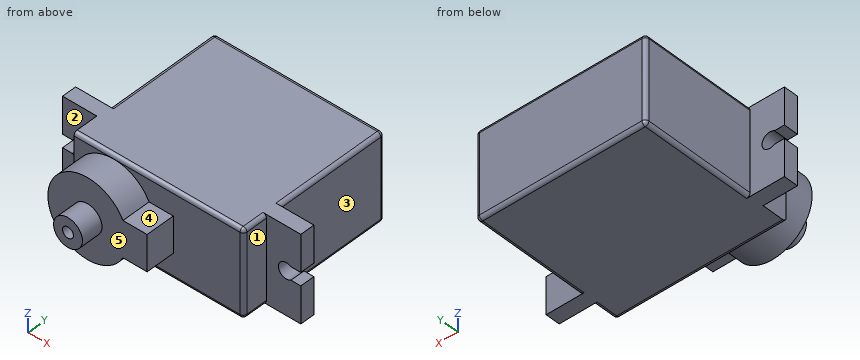
Autodesk Inventor part; units mm, degrees
ref_plane "YZ Plane" through (0, 0, 0) normal (1, 0, 0) x (0, 1, 0)
ref_plane "XZ Plane" through (0, 0, 0) normal (0, 1, 0) x (-1, 0, 0)
ref_plane "XY Plane" through (0, 0, 0) normal (0, 0, 1) x (1, 0, 0)
sketch "Sketch1" plane through (0, 0, 0) normal (0, 0, 1) x (1, 0, 0)
  line L0 (0, 0) -> (23.5, 0)
  line L1 (23.5, 0) -> (23.5, -21.5)
  line L2 (23.5, -21.5) -> (0, -21.5)
  line L3 (0, -21.5) -> (0, 0)
  dimension "d0" = 23.5
  dimension "d1" = 21.5
extrude "Extrusion1" add sketch "Sketch1" against normal blind 12
sketch "Sketch2" plane through (0, 0, 0) normal (0, 0, 1) x (1, 0, 0)
  line L0 (0, 0) -> (23.5, 0)
  line L1 (0, -21.5) -> (0, 0)
  line L2 (23.5, 0) -> (23.5, -21.5)
  line L3 (-4.75, -16) -> (28.25, -16)
  line L4 (28.25, -16) -> (28.25, -18)
  line L5 (28.25, -18) -> (-4.75, -18)
  line L6 (-4.75, -18) -> (-4.75, -16)
  dimension "d4" = 16
  dimension "d5" = 4.75
  dimension "d6" = 4.75
  dimension "d7" = 2
extrude "Extrusion2" add sketch "Sketch2" against normal blind 12 contours L3 L2 L5 L1 | L1 L5 L6 L3 | L3 L4 L5 L2
sketch "Sketch3" plane through (0, -21.5, 0) normal (0, -1, 0) x (1, 0, 0)
  line L0 (0, 0) -> (0, -12)
  circle A0 centre (5.5, -6) radius 5.5
  dimension "d10" = 5.5
  dimension "d11" = 11
extrude "Extrusion3" add sketch "Sketch3" along normal blind 4
sketch "Sketch4" plane through (5.5, -25.5, -6) normal (0, -1, 0) x (1, 0, 0)
  circle A0 centre (0, 0) radius 5.5
  line L0 (4.8288, 2.5) -> (8.25, 2.5)
  line L1 (8.25, 2.5) -> (8.25, -2.5)
  line L2 (8.25, -2.5) -> (4.8288, -2.5)
  line L3 (4.8288, -2.5) -> (4.8288, 2.5)
  point P0 (-5.5, 6)
  point P1 (8.25, 0)
  dimension "d15" = 5
  dimension "d17" = 8.25
extrude "Extrusion4" add sketch "Sketch4" against normal blind 4 contours A0 L2 L3 L0 | A0 L0 L1 L2 picked at (4.9626, -0.5673)
sketch "Sketch5" plane through (0, -25.5, 0) normal (0, -1, 0) x (1, 0, 0)
  arc A0 (10.399, -3.5) -> (10.399, -8.5) centre (5.5, -6) ccw
  circle A1 centre (5.5, -6) radius 2
  point P0 (0, 0)
  dimension "d20" = 4
extrude "Extrusion5" add sketch "Sketch5" along normal blind 3
sketch "Sketch6" plane through (-4.75, -18, 0) normal (0, -1, 0) x (1, 0, 0)
  line L0 (4.75, 0) -> (4.75, -12)
  line L1 (0, 0) -> (0, -12)
  line L2 (28.25, -12) -> (28.25, 0)
  line L3 (33, -12) -> (28.25, -12)
  line L4 (33, 0) -> (33, -12)
  line L5 (33, 0) -> (28.25, 0)
  circle A0 centre (2, -6) radius 1.1
  circle A1 centre (31, -6) radius 1.1
  line L6 (-3.3152, -5.1) -> (1.5271, -5.1)
  line L7 (1.5271, -5.1) -> (1.5271, -6.9)
  line L8 (1.5271, -6.9) -> (-3.3152, -6.9)
  line L9 (-3.3152, -6.9) -> (-3.3152, -5.1)
  line L10 (31.5226, -5.1) -> (37.6277, -5.1)
  line L11 (37.6277, -5.1) -> (37.6277, -6.9)
  line L12 (37.6277, -6.9) -> (31.5226, -6.9)
  line L13 (31.5226, -6.9) -> (31.5226, -5.1)
  point P0 (4.75, -6)
  point P1 (1.5271, -6)
  point P2 (28.25, -6)
  point P3 (31.5226, -6)
  dimension "d24" = 2.2
  dimension "d26" = 2
  dimension "d27" = 2
  dimension "d28" = 2.2
  dimension "d29" = 1.8
  dimension "d30" = 1.8
extrude "Extrusion6" cut sketch "Sketch6" against normal through all contours L6 A0 L8 L1 | L1 L8 L9 L6 | L6 L7 L8 A0 | A0 L8 L7 L6 | L12 A1 L10 L4 | L4 L10 L11 L12 | L12 L13 L10 A1 | A1 L10 L13 L12
fillet "Fillet1" radius 0.5 13 edges at (0, -8, -12) (23.5, -8, -12) (11.75, 0, -12) (11.75, 0, 0) (0, 0, -6) (23.5, 0, -6) (0, -8, 0) (23.5, -8, 0) (23.5, -19.75, 0) (23.5, -21.5, -6) (23.5, -19.75, -12) (11.75, -21.5, -12) (11.75, -21.5, 0)
sketch "Sketch7" plane through (5.5, -28.5, -6) normal (0, -1, 0) x (1, 0, 0)
  circle A0 centre (0, 0) radius 2
  point P0 (-5.5, 6)
hole "Hole1" at (5.5, -28.5, -6) direction (0, 1, 0) diameter 1.5 depth 8 tip angle 118
equation "\"d6\" = d5"
properties part number "Servo Motor"
Work out the finished part from the listing and answer in its coordinate system (mm). Face numbers are marked on the shaded views. A direction names the side the tool comes from. Coordinates: 2 decimals unless noted, no trailing zeros. Write each loop counter-clockwise with the first axis right and the second up, starting at its lowest first coordinate (ties: lowest second). Pieces come first, ordered by that corner, then holes. Notation, with made-up numbers: M 73.25,-15.75 L 92.25,-15.75 A18 ccw 92.25,8.25 Z; hole C 22.25,49.25 d6. An arc over 180 degrees is marked long. Write item = value, one per line.
1. Flat-ended cylindrical pins translate along their axes: pin 1 (2 mm diameter, centred on x = 7.5, y = -12.5, fed in from +Z); pin 2 (2 mm diameter, centred on y = -3.5, z = -3.5, fed in from +X); pin 3 (2 mm diameter, centred on x = 0, y = -25, fed in from +Z); pin 4 (6 mm diameter, centred on x = 27, z = -5.5, fed in from -Y). Find the tip coordinate at first contact, or state that the pin passes through.
Solution:
pin_1 = 0
pin_2 = 23.5
pin_3 = -2.84
pin_4 = -18
2. The part is cut by section C-C (x = 22). Determine the outline of the cut face in (y, z).
Solution:
outline = M -21.5,-11.5 A0.5 ccw -21,-12 L -0.5,-12 A0.5 ccw 0,-11.5 L 0,-0.5 A0.5 ccw -0.5,0 L -21,0 A0.5 ccw -21.5,-0.5 Z
3. The part is cut by section D-D (z = -4.5). Determine the outline of the cut face in (x, y).
Solution:
outline = M -4.75,-18 L 0,-18 L 0,-21.5 L 0.21,-21.5 L 0.21,-25.5 L 4.18,-25.5 L 4.18,-28.5 L 6.82,-28.5 L 6.82,-25.5 L 13.75,-25.5 L 13.75,-21.5 L 23,-21.5 A0.5 ccw 23.5,-21 L 23.5,-18 L 28.25,-18 L 28.25,-16 L 23.5,-16 L 23.5,-0.5 A0.5 ccw 23,0 L 0.5,0 A0.5 ccw 0,-0.5 L 0,-16 L -4.75,-16 Z
4. Straight lines are drawn through the part: line 1 (X direction, y = -23.75, z = -6); line 2 (Z direction, x = 26.25, y = -17.15); line 3 (X direction, y = -9.5, z = -1). For each, find the intervals that lie inside material, in ascending order. Write a range as from..to.
Solution:
line_1 = 0..4.75, 6.25..13.75
line_2 = -12..-7.1, -4.9..0
line_3 = 0..23.5
5. The part is cut by section A-A (x = 26.25). Determine the outline of the cut face in (y, z).
Solution:
outline = M -18,-12 L -16,-12 L -16,-7.1 L -18,-7.1 Z; M -18,-4.9 L -16,-4.9 L -16,0 L -18,0 Z
6. The part is cut by section B-B (y = -17.25). Determine the outline of the cut face in (x, z).
Solution:
outline = M -4.75,-12 L 28.25,-12 L 28.25,-6.9 L 26.88,-6.9 A1.1 cw long 26.88,-5.1 L 28.25,-5.1 L 28.25,0 L -4.75,0 L -4.75,-5.1 L -3.38,-5.1 A1.1 cw long -3.38,-6.9 L -4.75,-6.9 Z
7. For the marked faces 1, 2, 3, 4 and 5, determine the directions among +Z, -Z, +X, -X, +Y, -Y from which every point of the face is accessible in a straight line to the end or side of a thin tool.
Solution:
face_1 = +Z, -Z, +X, -Y
face_2 = +Z, -Z, -X, -Y
face_3 = +Z, -Z, +X, +Y
face_4 = +Z, +X, -Y
face_5 = -Y
